from build123d import *

# Parameters (mm, degrees)
F0_W     = 38
F0_H     = 17
F1_DEPTH = 15
F3_D     = 11
F5_D     = 5


with BuildPart() as f1:
    # F0 (on Top) → F1 (new body)
    with BuildSketch(Plane.XY):
        Rectangle(F0_W, F0_H)
    extrude(amount=F1_DEPTH)

    # F3 (through all)
    with Locations(Plane(origin=(0, 0, 0), x_dir=(1, 0, 0), z_dir=(0, 0, -1))):
        with Locations((0, 0)):
            Hole(F3_D / 2)

    # F5 (through all)
    with Locations(Plane.XZ.offset(8.5)):
        with Locations((-12, 7.5), (11.998904, 7.270673)):
            Hole(F5_D / 2)


solid = f1.part
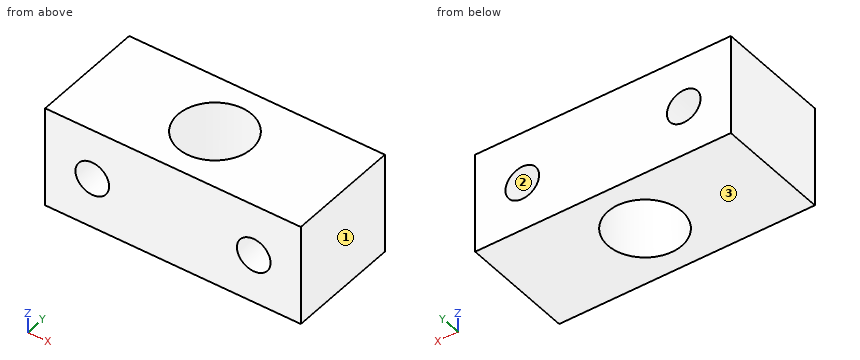
Input: part model. Units: mm. Frame: model coordinates. Face numbers are marked on the shaded views. Coordinates: 2 decimals unless noted, no trailing zeros. Order: outer loops, then holes, each group sorted by start corner. A loop starts at its lowest first (then second) coordinate and runs counter-clockwise, first axis right, second up. Notation, with made-up numbers: M -6.75,36 L 25.25,36 A34 ccw 25.25,67 Z; hole C 47.25,-35.5 d9. An arc over 180 degrees is marked long. Answer in a Markdown table with one row per item.
(1) Section query C-C, the plane y = 3.5. Output: boundary loops of the cut face in (x, z).
Numbers:
| item | result |
|---|---|
| outline | M -19,0 L -4.24,0 L -4.24,15 L -19,15 Z; M 4.24,0 L 19,0 L 19,15 L 4.24,15 Z; hole C -12,7.5 d5; hole C 12,7.27 d5 |
(2) Draft query along X for the marked faces 1, 2 and 3. Return one class per face: pulls with the +X half, pulls with the -X half, needs draft (parallel to the pull), parting line crosses it, or undercut.
Numbers:
| item | result |
|---|---|
| face 1 | pulls with the +X half |
| face 2 | undercut |
| face 3 | needs draft |
(3) Contact query for a flat-ended pin moving along its axis: pin 1 Ø4 at (x, z) = (-12, 7.5) entering from -Y. Output: stop coordinate, or through.
Numbers:
| item | result |
|---|---|
| pin 1 | passes through |
(4) Section query D-D, the plane z = 10.5. Output: boundary loops of the cut face in (x, y), plus the area to 3 significant figures.
Numbers:
| item | result |
|---|---|
| outline | M -19,-8.5 L 19,-8.5 L 19,8.5 L -19,8.5 Z; hole C 0,0 d11 |
| area | 551 mm^2 |
(5) Section query B-B, the plane z = 6.25. Output: boundary loops of the cut face in (x, y).
Numbers:
| item | result |
|---|---|
| outline | M -19,-8.5 L -14.17,-8.5 L -14.17,8.5 L -19,8.5 Z; M -9.83,-8.5 L 9.72,-8.5 L 9.72,8.5 L -9.83,8.5 Z; M 14.28,-8.5 L 19,-8.5 L 19,8.5 L 14.28,8.5 Z; hole C 0,0 d11 |
(6) Material intervals for line 1 (Y direction, x = 0, z = 4.25); line 2 (X direction, y = 1.75, z = 9.25); line 3 (X direction, y = 0.25, z = 11.75), sorted ascending. Write a range as [from, to].
Numbers:
| item | result |
|---|---|
| line 1 | y = [-8.5, -5.5], [5.5, 8.5] |
| line 2 | x = [-19, -13.79], [-10.21, -5.21], [5.21, 10.47], [13.53, 19] |
| line 3 | x = [-19, -5.49], [5.49, 19] |
(7) Section query A-A, the plane x = -12. Output: boundary loops of the cut face in (y, z).
Numbers:
| item | result |
|---|---|
| outline | M -8.5,0 L 8.5,0 L 8.5,5 L -8.5,5 Z; M -8.5,10 L 8.5,10 L 8.5,15 L -8.5,15 Z |
